Input: part model. Units: mm. Frame: model coordinates. Face numbers are marked on the shaded views. A direction names the side the tool comes from. Round coordinates to 2 decimals unless told otherwise and drop trailing zeros. Loops run counter-clockwise (first coordinate to the right, second up) from the corner with the lowest first, then second, coordinate; pieces in that order, holes last. Notation, with made-up numbers: (-6, 55.5) -> (28, 55.5) arc R18 cw to (28, 71.5) -> close; hole circle Ø9 at (33, 55.25). An arc over 180 degrees is marked (long way). Answer in a Markdown table with one row per item. Add a question column.
Q1. Ray query, L1, parallel to Z at x = -12.25, y = -14; L2, parallel to Y at x = -2, z = 1; L3, parallel to X at y = -17.7, z = 5. Return the intervals inside material, ascending. Write a range as from..to.
Q2. Pin query (flat end, axial travel): pin 1 (5 mm diameter, centred on x = 3.5, y = -13, fed in from -Z); pin 2 (2 mm diameter, centred on x = -1, z = 6, fed in from +Y); pin 3 (5 mm diameter, centred on x = 1.5, y = -5.5, fed in from -Z). Return the tip coordinate at first contact, or that it passes through.
Q3. Section A-A, the plane z = 0.5. Output: boundary loops of the cut face in (x, y), and give its area (3 significant figures).
Q4. Section B-B, the plane y = -15. Output: boundary loops of the cut face in (x, z).
Q5. Reachability of the marked faces 1, 2, 3 and 4 from +Z, -Z, +X, -X, +Y, -Y: full face, straight path, thin tool, end or side. Return the list, or none.
Q6. Section C-C, the plane x = 4.5. Output: boundary loops of the cut face in (y, z), and give its area (3 significant figures).
Q7. Mould query, pull axis Z, two halves, no side actions, for the marked faces 5, 6 and 7. Classes: pulls with the +Z half, pulls with the -Z half, needs draft (parallel to the pull), parting line crosses it, or undercut.
Q8. Section D-D, the plane z = -7.5. Output: boundary loops of the cut face in (x, y), and give its area (3 significant figures).
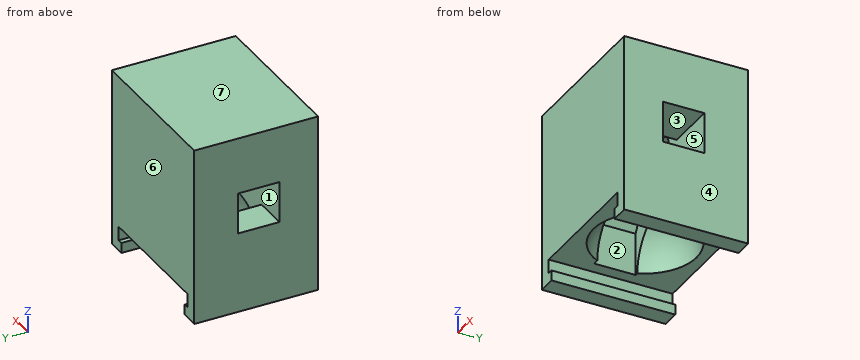
```python
from build123d import *

# Parameters (mm, degrees)
F0_W     = 5
F0_H     = 8
F0_H_2   = 11
F0_W_2   = 2.5
F0_H_3   = 2.7
F0_W_3   = 1.5
F1_DEPTH = 24
F4_START = 8.5
F4_DEPTH = 8
F6_START = -4
F6_DEPTH = 17


with BuildPart() as f1:
    # F0 (on Front) → F1 (new body)
    with BuildSketch(Plane.XZ):
        with Locations((-12.5, 0)):
            Rectangle(F0_W, F0_H)
        with Locations((12.5, 9.5)):
            Rectangle(F0_W, F0_H_2)
        with BuildLine():
            Line((10, 4), (10, 15))
            Line((10, 15), (0, 15))
            Line((0, 15), (0, 13))
            ThreePointArc((0, 13), (2.9140227369, 12.5151906314), (5.5141020242, 11.1129936642))
            Line((5.5141020242, 11.1129936642), (3.727430731, 6.2041546301))
            Line((3.727430731, 6.2041546301), (5, 4))
            Line((5, 4), (8.5, 4))
            Line((8.5, 4), (10, 4))
        make_face()
        Polygon((0, 0), (0, 1.9517640748), (-8.5, -4), (0, -4), align=None)
        Polygon((15, -19.7), (15, -17.7), (12.5, -17.7), (11.5, -17.7), (11.5, -19.7), align=None)
        Polygon((0, -4), (8.5, -4), (0, 1.9517640748), (0, 0), align=None)
        Polygon((10, -6.7414640249), (10, -4), (8.5, -4), align=None)
        with BuildLine():
            Line((0, 13), (0, 15))
            Line((0, 15), (-10, 15))
            Line((-10, 15), (-10, 4))
            Line((-10, 4), (-8.5, 4))
            Line((-8.5, 4), (-5, 4))
            Line((-5, 4), (-3.727430731, 6.2041546301))
            Line((-3.727430731, 6.2041546301), (-5.5141020242, 11.1129936642))
            ThreePointArc((-5.5141020242, 11.1129936642), (-2.9140227369, 12.5151906314), (0, 13))
        make_face()
        with Locations((13.75, -16.35)):
            Rectangle(F0_W_2, F0_H_3)
        Polygon((10, -6.7414640249), (8.5, -4), (0, -4), (0, -15), (10, -15), align=None)
        Polygon((15, -15), (15, -4), (10, -4), (10, -6.7414640249), (10, -15), (12.5, -15), align=None)
        Polygon((0, -15), (0, -4), (-8.5, -4), (-10, -6.7414640249), (-10, -15), align=None)
        with BuildLine():
            ThreePointArc((5.5141020242, 11.1129936642), (2.9140227369, 12.5151906314), (0, 13))
            Line((0, 13), (0, 4))
            Line((0, 4), (2.9251840539, 4))
            Line((2.9251840539, 4), (3.727430731, 6.2041546301))
            Line((3.727430731, 6.2041546301), (5.5141020242, 11.1129936642))
        make_face()
        with BuildLine():
            Line((0, 4), (0, 13))
            ThreePointArc((0, 13), (-2.9140227369, 12.5151906314), (-5.5141020242, 11.1129936642))
            Line((-5.5141020242, 11.1129936642), (-3.727430731, 6.2041546301))
            Line((-3.727430731, 6.2041546301), (-2.9251840539, 4))
            Line((-2.9251840539, 4), (0, 4))
        make_face()
        with Locations((12.5, 0)):
            Rectangle(F0_W, F0_H)
        Polygon((-11.5, -19.7), (-11.5, -17.7), (-12.5, -17.7), (-15, -17.7), (-15, -19.7), align=None)
        with Locations((9.25, 0)):
            Rectangle(F0_W_3, F0_H)
        Polygon((-5, 4), (-2.9251840539, 4), (-3.727430731, 6.2041546301), align=None)
        with Locations((-13.75, -16.35)):
            Rectangle(F0_W_2, F0_H_3)
        with Locations((-12.5, 9.5)):
            Rectangle(F0_W, F0_H_2)
        Polygon((-8.5, -4), (-10, -4), (-10, -6.7414640249), align=None)
        Polygon((8.5, -4), (8.5, 4), (5, 4), (2.9251840539, 4), (0, 1.9517640748), align=None)
        Polygon((-5, 4), (-8.5, 4), (-8.5, -4), (0, 1.9517640748), (-2.9251840539, 4), align=None)
        Polygon((2.9251840539, 4), (5, 4), (3.727430731, 6.2041546301), align=None)
        Polygon((2.9251840539, 4), (0, 4), (0, 1.9517640748), align=None)
        Polygon((0, 1.9517640748), (0, 4), (-2.9251840539, 4), align=None)
        with Locations((-9.25, 0)):
            Rectangle(F0_W_3, F0_H)
        Polygon((-10, -6.7414640249), (-10, -4), (-15, -4), (-15, -15), (-12.5, -15), (-10, -15), align=None)
    extrude(amount=F1_DEPTH)

    # F2 (on face) → F3 (revolve, cut)
    with BuildSketch(Plane(origin=(0, 0, -15), x_dir=(1, 0, 0), z_dir=(0, 0, -1))):
        with BuildLine():
            ThreePointArc((0, 22), (-10, 12), (0, 2))
            Line((0, 2), (0, 12))
            Line((0, 12), (0, 22))
        make_face()
    revolve(axis=Axis((0, -6, -15), (0, -1, 0)), mode=Mode.SUBTRACT)

    # F0 (on Front) → F4 (cut)
    with BuildSketch(Plane.XZ.offset(F4_START)):
        Polygon((10, -6.7414640249), (8.5, -4), (0, -4), (0, -15), (10, -15), align=None)
        Polygon((0, -4), (8.5, -4), (0, 1.9517640748), (0, 0), align=None)
        Polygon((8.5, -4), (8.5, 4), (5, 4), (2.9251840539, 4), (0, 1.9517640748), align=None)
        Polygon((2.9251840539, 4), (0, 4), (0, 1.9517640748), align=None)
        Polygon((0, 1.9517640748), (0, 4), (-2.9251840539, 4), align=None)
        Polygon((0, 0), (0, 1.9517640748), (-8.5, -4), (0, -4), align=None)
        Polygon((-5, 4), (-8.5, 4), (-8.5, -4), (0, 1.9517640748), (-2.9251840539, 4), align=None)
        with Locations((-9.25, 0)):
            Rectangle(F0_W_3, F0_H)
        with Locations((-12.5, 0)):
            Rectangle(F0_W, F0_H)
        with Locations((9.25, 0)):
            Rectangle(F0_W_3, F0_H)
        with Locations((12.5, 0)):
            Rectangle(F0_W, F0_H)
        with BuildLine():
            ThreePointArc((5.5141020242, 11.1129936642), (2.9140227369, 12.5151906314), (0, 13))
            Line((0, 13), (0, 4))
            Line((0, 4), (2.9251840539, 4))
            Line((2.9251840539, 4), (3.727430731, 6.2041546301))
            Line((3.727430731, 6.2041546301), (5.5141020242, 11.1129936642))
        make_face()
        with BuildLine():
            Line((0, 4), (0, 13))
            ThreePointArc((0, 13), (-2.9140227369, 12.5151906314), (-5.5141020242, 11.1129936642))
            Line((-5.5141020242, 11.1129936642), (-3.727430731, 6.2041546301))
            Line((-3.727430731, 6.2041546301), (-2.9251840539, 4))
            Line((-2.9251840539, 4), (0, 4))
        make_face()
        Polygon((0, -15), (0, -4), (-8.5, -4), (-10, -6.7414640249), (-10, -15), align=None)
        Polygon((2.9251840539, 4), (5, 4), (3.727430731, 6.2041546301), align=None)
        Polygon((-5, 4), (-2.9251840539, 4), (-3.727430731, 6.2041546301), align=None)
    extrude(amount=F4_DEPTH, mode=Mode.SUBTRACT)

    # F5 (on face) → F6 (cut)
    with BuildSketch(Plane(origin=(0, 0, 0), x_dir=(-1, 0, 0), z_dir=(0, 1, 0)).offset(F6_START)):
        with BuildLine():
            ThreePointArc((0, 3), (1.4142135624, 3.5857864376), (2, 5))
            ThreePointArc((2, 5), (-1.4142135624, 6.4142135624), (0, 3))
        make_face()
    extrude(amount=-F6_DEPTH, mode=Mode.SUBTRACT)


solid = f1.part
```
Answer block:
| question | item | result |
|---|---|---|
| 1 | L1 | -19.7..-17.7, -15..-4, 4..15 |
| 1 | L2 | -24..-16.5, -8.5..0 |
| 1 | L3 | -15..-2, 2..15 |
| 2 | pin 1 | z = 4 |
| 2 | pin 2 | y = 0 |
| 2 | pin 3 | z = -11.01 |
| 3 | outline | (-15, -24) -> (15, -24) -> (15, -16.5) -> (-15, -16.5) -> close; (-15, -8.5) -> (15, -8.5) -> (15, 0) -> (-15, 0) -> close |
| 3 | area | 480 mm^2 |
| 4 | outline | (-15, -19.7) -> (-11.5, -19.7) -> (-11.5, -17.7) -> (-12.5, -17.7) -> (-12.5, -15) -> (-10, -15) -> (-10, -6.74) -> (-8.5, -4) -> (-15, -4) -> close; (-15, 4) -> (-5, 4) -> (-3.73, 6.2) -> (-5.51, 11.11) arc R9 cw to (5.51, 11.11) -> (3.73, 6.2) -> (5, 4) -> (15, 4) -> (15, 15) -> (-15, 15) -> close; (8.5, -4) -> (10, -6.74) -> (10, -15) -> (12.5, -15) -> (12.5, -17.7) -> (11.5, -17.7) -> (11.5, -19.7) -> (15, -19.7) -> (15, -4) -> close |
| 5 | face 1 | none |
| 5 | face 2 | -Z |
| 5 | face 3 | +X, -X |
| 5 | face 4 | +Z, -Z, +X, +Y, -Y |
| 6 | outline | (-24, -15) -> (-20.93, -15) arc R8.93 cw to (-16.5, -7.29) -> (-16.5, 4.87) -> (-8.5, 4.87) -> (-8.5, -6.78) arc R8.93 cw to (-3.07, -15) -> (0, -15) -> (0, 15) -> (-24, 15) -> close; hole (-16.5, 8.33) -> (-8.5, 8.33) -> (-8.5, 11.79) -> (-16.5, 11.79) -> close |
| 6 | area | 477 mm^2 |
| 7 | face 5 | undercut |
| 7 | face 6 | needs draft |
| 7 | face 7 | pulls with the +Z half |
| 8 | outline | (-15, -24) -> (15, -24) -> (15, 0) -> (-15, 0) -> close; hole (-10, -16.5) -> (-4.85, -16.5) arc R6.61 ccw to (4.85, -16.5) -> (10, -16.5) -> (10, -8.5) -> (5.61, -8.5) arc R6.61 ccw to (-5.61, -8.5) -> (-10, -8.5) -> close |
| 8 | area | 521 mm^2 |
